Design review of the part built by this model. Coordinates are the model's own, in mm. Coordinates: 2 decimals unless noted, no trailing zeros. Loops run counter-clockwise (first coordinate to the right, second up) from the corner with the lowest first, then second, coordinate; pieces in that order, holes last. Notation, with made-up numbers: M 9.5,79.5 L 38.5,79.5 A26 ccw 38.5,96.5 Z; hole C 5,33 d1. An arc over 180 degrees is marked long. Write item = value, one per line. Start each with the question number.
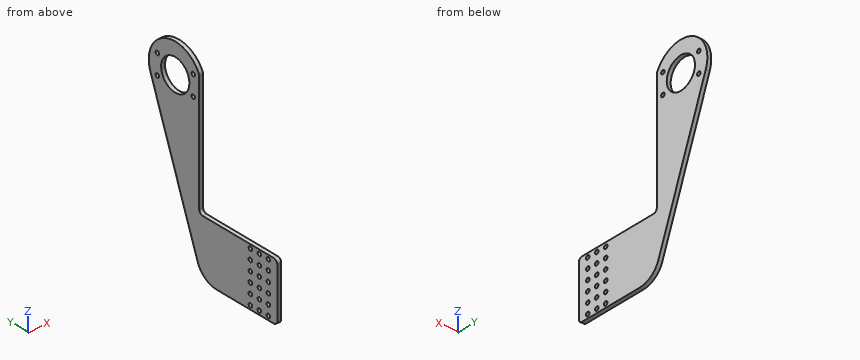
Autodesk Inventor part; units mm, degrees
ref_plane "YZ Plane" through (0, 0, 0) normal (1, 0, 0) x (0, 1, 0)
ref_plane "XZ Plane" through (0, 0, 0) normal (0, 1, 0) x (-1, 0, 0)
ref_plane "XY Plane" through (0, 0, 0) normal (0, 0, 1) x (1, 0, 0)
sketch "Esboço1" plane through (0, 0, 0) normal (1, 0, 0) x (0, 1, 0)
  line L0 (0, 0) -> (50.8, 0)
  line L1 (50.8, 0) -> (50.8, -86.2)
  line L2 (50.8, -86.2) -> (0, -86.2)
  line L3 (0, -86.2) -> (0, 0)
  dimension "d0" = 50.8
  dimension "d1" = 86.2
extrude "Extrusão1" add sketch "Esboço1" along normal blind 5
sketch "Esboço2" plane through (5, 0, 0) normal (1, 0, 0) x (0, 0, -1)
  circle A0 centre (5, 12.7) radius 2.5
  circle A1 centre (5, 25.4) radius 2.5
  circle A2 centre (5, 38.1) radius 2.5
  line L0 (0, 50.8) -> (0, 0)
  line L1 (86.2, 50.8) -> (0, 50.8)
  line L2 (0, 0) -> (86.2, 0)
  dimension "d4" = 5
  dimension "d5" = 5
  dimension "d6" = 5
  dimension "d7" = 5
  dimension "d8" = 5
  dimension "d9" = 5
  dimension "d10" = 12.7
  dimension "d11" = 12.7
  dimension "d12" = 12.7
extrude "Extrusão2" cut sketch "Esboço2" against normal blind 6
pattern_linear "Padrão retangular1" count 7 spacing 12.7 along (0, 0, -1) of "Extrusão2"
sketch "Esboço3" plane through (0, 0, 0) normal (-1, 0, 0) x (0, 0, 1)
  line L0 (0, 50.8) -> (0, 0)
  line L1 (0, 0) -> (-86.2, 0)
  line L2 (0, 50.8) -> (-50.8, 50.8)
  line L3 (-50.8, 50.8) -> (-50.8, 0)
  line L4 (-50.8, 0) -> (0, 0)
  line L5 (0, 0) -> (0, 50.8)
  circle A0 centre (-55.8, 25.4) radius 2.5
  dimension "d19" = 5
extrude "Extrusão3" cut sketch "Esboço3" against normal blind 10 contours L0 L1 L3 L2
sketch "Esboço4" plane through (5, 0, 0) normal (1, 0, 0) x (0, 0, -1)
  line L0 (86.2, 0) -> (86.2, 50.8)
  line L1 (86.2, 50.8) -> (124.3, 50.8)
  line L2 (124.3, 50.8) -> (124.3, 0)
  line L3 (124.3, 0) -> (86.2, 0)
  line L4 (86.2, 0) -> (86.2, 50.8)
  circle A0 centre (93.9, 25.4) radius 2.5
  circle A1 centre (93.9, 38.1) radius 2.5
  circle A2 centre (106.6, 38.1) radius 2.5
  circle A3 centre (119.3, 38.1) radius 2.5
  circle A4 centre (119.3, 25.4) radius 2.5
  circle A5 centre (106.6, 25.4) radius 2.5
  circle A6 centre (93.9, 12.7) radius 2.5
  circle A7 centre (106.6, 12.7) radius 2.5
  circle A8 centre (119.3, 12.7) radius 2.5
  point P0 (0, 0)
  dimension "d22" = 5
  dimension "d23" = 50.8
extrude "Extrusão4" add sketch "Esboço4" against normal blind 5
sketch "Esboço7" plane through (5, 0, 0) normal (1, 0, 0) x (0, 0, -1)
  line L0 (124.3, 50.8) -> (50.8, 50.8)
  line L1 (124.3, 50.8) -> (124.3, 85.9607)
  circle A0 centre (95.7, 85.9607) radius 11.25
  circle A1 centre (-89.125, 144.496) radius 17.5
  circle A2 centre (95.7, 111.3607) radius 2.0193
  circle A3 centre (77.7395, 103.9212) radius 2.0193
  circle A4 centre (95.7, 60.5607) radius 2.0193
  circle A5 centre (113.6605, 68.0002) radius 2.0193
  circle A6 centre (-101.825, 169.896) radius 2.5
  circle A7 centre (-76.425, 169.896) radius 2.5
  circle A8 centre (-76.425, 119.096) radius 2.5
  circle A9 centre (-101.825, 119.096) radius 2.5
  arc A10 (-76.1735, 179.6885) -> (-105.0332, 110.5375) centre (-89.125, 144.496) ccw
  arc A11 (124.3, 85.9607) -> (105.5776, 112.8008) centre (95.7, 85.9607) ccw
  line L2 (50.8, 0) -> (50.8, 50.8)
  line L3 (50.8, 50.8) -> (50.8, 110.5375)
  line L4 (50.8, 110.5375) -> (-105.0332, 110.5375)
  line L5 (54.784, 109.5375) -> (24.05, 109.5375)
  line L6 (-76.1735, 179.6885) -> (105.5776, 112.8008)
  circle A12 centre (-89.125, 144.496) radius 20
  circle A13 centre (95.7, 85.9607) radius 14.25
  point P0 (0, 0)
  dimension "d36" = 75
  dimension "d37" = 1
  dimension "d38" = 40
  dimension "d39" = 28.5
extrude "Extrusão6" add sketch "Esboço7" against normal blind 5 contours L0 L3 L4 A10 L6 A11 L1
fillet "Arredondamento1" radius 5 4 edges at (2.5, 110.5375, -50.8) (2.5, 110.5375, 105.0332) (2.5, 0, -50.8) (2.5, 0, -124.3)
sketch "Esboço8" plane through (0, 0, 0) normal (-1, 0, 0) x (0, 0, 1)
  circle A0 centre (-95.7, 85.9607) radius 14.25
  circle A1 centre (-113.6605, 68.0002) radius 2.0193
  circle A2 centre (-95.7, 60.5607) radius 2.0193
  circle A3 centre (-95.7, 111.3607) radius 2.0193
  circle A4 centre (-77.7395, 103.9212) radius 2.0193
  point P0 (0, 0)
extrude "Extrusão7" add sketch "Esboço8" against normal blind 5
equation "\"d8\" = d7"
equation "\"d9\" = d8"
equation "\"d11\" = d10"
equation "\"d12\" = d11"
properties part number "CHAPA FIXAÇÃO DIREITA 2"
(1) Take a section at B-B (z = -81.2). State the section outline as (x, y) points, plus the area to 3 significant figures.
(2) To check wall thickness, follow L1, parallel to Y at x = 4, z = -55.8; L2, parallel to Y at x = 2.75, z = -106.6; L3, parallel to Z at x = 4.85, y = 72. State the ranges of each line that lie inside material, in increasing order.
(3) Insertion check: pin 1 (6 mm diameter, centred on y = 38.1, z = -81.2, fed in from -X); pin 2 (1.5 mm diameter, centred on x = 4.5, z = -14, fed in from -Y); pin 3 (2.5 mm diameter, centred on x = 3.5, y = 74.5, fed in from +Z). Each pin has a flat end and moves straight along its axis. Give the tip position at first contact, or say it passes through.
(4) Take a section at C-C (x = 2.7). Give the number of separate pieces and of enclosed holes in the cut face, plus the area to 3 significant figures.
(5) Take a section at D-D (y = 83). State the section outline as (x, z) points, plus the area to 4 significant figures.
(6) Take a section at A-A (y = 25.4). State the section outline as (x, z) points.
Results list:
q1.outline = M 0,0 L 5,0 L 5,10.2 L 0,10.2 Z; M 0,15.2 L 5,15.2 L 5,22.9 L 0,22.9 Z; M 0,27.9 L 5,27.9 L 5,35.6 L 0,35.6 Z; M 0,40.6 L 5,40.6 L 5,121.77 L 0,121.77 Z
q1.area = 534 mm^2
q2.L1 = 0 to 10.2, 15.2 to 22.9, 27.9 to 35.6, 40.6 to 131.12
q2.L2 = 0 to 10.2, 15.2 to 22.9, 27.9 to 35.6, 40.6 to 112.4
q2.L3 = -124.3 to -50.8
q3.pin_1 = 0
q3.pin_2 = 110.54
q3.pin_3 = -50.8
q4.separate_pieces = 1
q4.enclosed_holes = 23
q4.area = 15,900 mm^2
q5.outline = M 0,-124.3 L 5,-124.3 L 5,-50.8 L 0,-50.8 Z
q5.area = 367.5 mm^2
q6.outline = M 0,-124.3 L 5,-124.3 L 5,-121.8 L 0,-121.8 Z; M 0,-116.8 L 5,-116.8 L 5,-109.1 L 0,-109.1 Z; M 0,-104.1 L 5,-104.1 L 5,-96.4 L 0,-96.4 Z; M 0,-91.4 L 5,-91.4 L 5,-83.7 L 0,-83.7 Z; M 0,-78.7 L 5,-78.7 L 5,-71 L 0,-71 Z; M 0,-66 L 5,-66 L 5,-58.3 L 0,-58.3 Z; M 0,-53.3 L 5,-53.3 L 5,-50.8 L 0,-50.8 Z
